```python
from build123d import *

# Parameters (mm, degrees)
SM_BASE_FLANGE_1_DEPTH = 10
HOLE_WIZARD_M4_1_D     = 3.3


# Sheet-metal steps are written as plain solids
with BuildPart() as part:
    # Sketch 1 → 基体-法兰1 (new, symmetric)
    with BuildSketch(Plane.XY):
        with BuildLine():
            Line((0, 0), (-9, 0))
            ThreePointArc((-9, 0), (-9.707106781, -0.292893219), (-10, -1))
            Line((-10, -1), (-10, -55.5))
            Line((-10, -55.5), (-11.5, -55.5))
            Line((-11.5, -55.5), (-11.5, -1))
            ThreePointArc((-11.5, -1), (-10.767766953, 0.767766953), (-9, 1.5))
            Line((-9, 1.5), (0, 1.5))
            Line((0, 1.5), (0, 0))
        make_face()
    extrude(amount=SM_BASE_FLANGE_1_DEPTH, both=True)

    # M4 螺纹孔1 (through all)
    with Locations(Plane(origin=(0, 1.5, 0), x_dir=(1, 0, 0), z_dir=(0, 1, 0))):
        with Locations((-4, 5), (-4, -5)):
            Hole(HOLE_WIZARD_M4_1_D / 2)


solid = part.part
```
Work out the finished part from the listing and answer in its coordinate system (mm). A direction names the side the tool comes from. Round coordinates to 2 decimals unless told otherwise and drop trailing zeros. Order: outer loops, then holes, each group sorted by start corner. A loop starts at its lowest first (then second) coordinate and runs counter-clockwise, first axis right, second up.
Q1. A cutting plane is placed at D-D, the plane y = -25.5. Determine the outline of the cut face in (x, z), then the cut area to 3 significant figures.
Solution:
outline: (-11.5, -10) - (-10, -10) - (-10, 10) - (-11.5, 10) - close
area: 30.0 mm2
Q2. A cutting plane is placed at C-C, the plane z = 0. Determine the outline of the cut face in (x, y), then the cut area to 3 significant figures.
Solution:
outline: (-11.5, -55.5) - (-10, -55.5) - (-10, -1) arc R1 cw to (-9, 0) - (0, 0) - (0, 1.5) - (-9, 1.5) arc R2.5 ccw to (-11.5, -1) - close
area: 99.4 mm2
Q3. A tool of negligible diameter and unlimited length cuts with its end or side. For faces 1 (the flat face through (-11, -55.5, 0)), 2 (the flat face through (-10, -28, 0)), from which of +Z, -Z, +X, -X, +Y, -Y can it reach the whole face along a straight path? Write none if from no direction.
Solution:
face 1: +Z, -Z, +X, -X, -Y
face 2: +Z, -Z, +X, -Y
Q4. A cutting plane is placed at B-B, the plane x = -4. Determine the outline of the cut face in (y, z).
Solution:
outline: (0, -10) - (1.5, -10) - (1.5, -6.65) - (0, -6.65) - close; (0, -3.35) - (1.5, -3.35) - (1.5, 3.35) - (0, 3.35) - close; (0, 6.65) - (1.5, 6.65) - (1.5, 10) - (0, 10) - close
Q5. Find the intervals of material crossed by line 1 along Z through (x, y) = (-4, 0.95); line 2 along X through (y, z) = (-41.5, -7.25); line 3 along Y through (x, z) = (-7.5, -5.5), in increasing order.
Solution:
line 1: z = -10 to -6.65, -3.35 to 3.35, 6.65 to 10
line 2: x = -11.5 to -10
line 3: y = 0 to 1.5
Q6. A cutting plane is placed at A-A, the plane z = -5. Determine the outline of the cut face in (x, y), then the cut area to 3 significant figures.
Solution:
outline: (-11.5, -55.5) - (-10, -55.5) - (-10, -1) arc R1 cw to (-9, 0) - (-5.65, 0) - (-5.65, 1.5) - (-9, 1.5) arc R2.5 ccw to (-11.5, -1) - close; (-2.35, 0) - (0, 0) - (0, 1.5) - (-2.35, 1.5) - close
area: 94.4 mm2
Q7. The mould has two halves that part along X. Classify faces 3 (the cylindrical face through (-2.69, 0.74, 6)), 4 (the flat face through (-10.4, -20.5, -10)), 5 (the cylindrical face through (-9.699, -0.285, 0.14)): pulls with the +X half, pulls with the -X half, needs draft (parallel to the pull), parting line crosses it, or undercut.
Solution:
face 3: undercut
face 4: needs draft
face 5: pulls with the +X half
Q8. Given pin 1 Ø10 at (y, z) = (-45.5, 0.5) entering from +X; pin 2 Ø2 at (x, z) = (-6, 4) entering from -Y, each flat-ended and moving along its own axis, determine where each tip first touches the part or whether it passes through.
Solution:
pin 1: stops at x = -10
pin 2: stops at y = 0
